Autodesk Inventor part; units mm, degrees
ref_plane "YZ Plane" through (0, 0, 0) normal (1, 0, 0) x (0, 1, 0)
ref_plane "XZ Plane" through (0, 0, 0) normal (0, 1, 0) x (-1, 0, 0)
ref_plane "XY Plane" through (0, 0, 0) normal (0, 0, 1) x (1, 0, 0)
sketch "Sketch1" plane through (0, 0, 0) normal (0, 1, 0) x (-1, 0, 0)
  line L0 (15.5, 13) -> (-15.5, 13)
  line L1 (-15.5, 13) -> (-15.5, -13)
  line L2 (-15.5, -13) -> (15.5, -13)
  line L3 (15.5, -13) -> (15.5, 13)
  line L4 (15.5, 13) -> (-15.5, -13) construction
  line L5 (-15.5, 13) -> (15.5, -13) construction
  circle A0 centre (0, 0) radius 12
  circle A1 centre (12, 9.5) radius 1.8
  circle A2 centre (-12, -9.5) radius 1.8
  line L6 (18.75, -14.25) -> (-18.75, -14.25)
  line L7 (-18.75, -14.25) -> (-18.75, 14.25)
  line L8 (-18.75, 14.25) -> (18.75, 14.25)
  line L9 (18.75, 14.25) -> (18.75, -14.25)
  line L10 (18.75, -14.25) -> (-18.75, 14.25) construction
  line L11 (-18.75, -14.25) -> (18.75, 14.25) construction
  dimension "d0" = 31
  dimension "d1" = 26
  dimension "d2" = 24
  dimension "d7" = 3.6
  dimension "d8" = 9.5
  dimension "d9" = 12
  dimension "d10" = 3.6
  dimension "d11" = 9.5
  dimension "d12" = 12
  dimension "d16" = 37.5
  dimension "d17" = 28.5
extrude "Extrusion2" add sketch "Sketch1" along normal blind 4 contours L3 L2 L1 L0 | L6 L7 L8 L9
sketch "Sketch2" plane through (0, 4, 0) normal (0, 1, 0) x (1, 0, 0)
  line L0 (15.5, 13) -> (-15.5, 13)
  line L1 (-15.5, -13) -> (15.5, -13)
  line L2 (-18.75, -14.25) -> (18.75, -14.25)
  line L3 (18.75, -14.25) -> (18.75, 14.25)
  line L4 (18.75, 14.25) -> (-18.75, 14.25)
  line L5 (-18.75, 14.25) -> (-18.75, -14.25)
  circle A0 centre (0, 0) radius 12
  circle A1 centre (-12, -9.5) radius 1.8
  circle A2 centre (12, 9.5) radius 1.8
  line L6 (15.5, -13) -> (15.5, 13)
  line L7 (-15.5, 13) -> (-15.5, -13)
extrude "Extrusion3" cut sketch "Sketch2" against normal blind 1 contours L6 L1 L7 L0 | A0 | A1 | A2
fillet "Fillet2" radius 2 4 edges at (-15.5, 3.5, -13) (-15.5, 3.5, 13) (15.5, 3.5, 13) (15.5, 3.5, -13)
equation "\"d10\" = d7"
properties part number "inner clamp plate_3DPrint"
CAD build for the part. Positions are in the model's coordinates, mm. A direction names the side the tool comes from. Round coordinates to 2 decimals unless told otherwise and drop trailing zeros. Order: outer loops, then holes, each group sorted by start corner. A loop starts at its lowest first (then second) coordinate and runs counter-clockwise, first axis right, second up.
Item 1: Saw through at C-C on y = 2.6. Write the cut outline in (x, z).
Item 2: Probe line 1 along Z through (x, y) = (0, 1.05); line 2 along X through (y, z) = (1.65, -9.5); line 3 along X through (y, z) = (3.5, 11). List the from-to ranges inside material, lowest first.
Item 3: Tool access for faces 1 (the face through (14.93, 3.49, 12.4)), 2 (the face through (-11.61, 1.479, 11.257)): list every direction of +Z, -Z, +X, -X, +Y, -Y with a clear straight run to the whole face (end or side of a thin tool).
Item 4: Saw through at B-B on z = 0. Write the cut outline in (x, y), then the cut area to 3 significant figures.
Item 5: Mould opens along X. For faces 3 (the face through (-18.75, 2, 0)), 4 (the face through (-11, 3, -6)), 5 (the face through (0, 2, 14.25)) say: pulls with the +X half, pulls with the -X half, needs draft (parallel to the pull), parting line crosses it, or undercut.
Item 6: Saw through at D-D on z = -9. Write the cut outline in (x, y), then the cut area to 3 significant figures.
Item 7: Saw through at A-A on x = 0. Write the cut outline in (y, z), then the cut area to 3 significant figures.
Item 8: Pin check, flat tips, straight feed: pin 1 (4.5 mm diameter, centred on x = 12, z = -9.5, fed in from +Y); pin 2 (1 mm diameter, centred on x = 5, z = 9.5, fed in from -Y). Stop position of each tip, or through.
Reported:
1. outline: (-18.75, -14.25) - (18.75, -14.25) - (18.75, 14.25) - (-18.75, 14.25) - close; hole circle Ø3.6 at (-12, 9.5); hole circle Ø24 at (0, 0); hole circle Ø3.6 at (12, -9.5)
2. line 1: z = -14.25 to -12, 12 to 14.25
2. line 2: x = -18.75 to -7.33, 7.33 to 10.2, 13.8 to 18.75
2. line 3: x = -18.75 to -15.5, 15.5 to 18.75
3. face 1: +Y
3. face 2: +Y, -Y
4. outline: (-18.75, 0) - (-12, 0) - (-12, 3) - (-15.5, 3) - (-15.5, 4) - (-18.75, 4) - close; (12, 0) - (18.75, 0) - (18.75, 4) - (15.5, 4) - (15.5, 3) - (12, 3) - close
4. area: 47.0 mm2
5. face 3: pulls with the -X half
5. face 4: undercut
5. face 5: needs draft
6. outline: (-18.75, 0) - (-7.94, 0) - (-7.94, 3) - (-15.5, 3) - (-15.5, 4) - (-18.75, 4) - close; (7.94, 0) - (10.27, 0) - (10.27, 3) - (7.94, 3) - close; (13.73, 0) - (18.75, 0) - (18.75, 4) - (15.5, 4) - (15.5, 3) - (13.73, 3) - close
6. area: 61.0 mm2
7. outline: (0, -14.25) - (4, -14.25) - (4, -13) - (3, -13) - (3, -12) - (0, -12) - close; (0, 12) - (3, 12) - (3, 13) - (4, 13) - (4, 14.25) - (0, 14.25) - close
7. area: 16.0 mm2
8. pin 1: stops at y = 3
8. pin 2: passes through
